```python
from build123d import *
from build123d.topology import SkipClean

# Parameters (mm, degrees)
BOSS_EXTRUDE1_DEPTH      = 3
BOSS_EXTRUDE1_DEPTH_BACK = 1.5
SKETCH1_R                = 8
SKETCH2_W                = 16
SKETCH2_H                = 30
BOSS_EXTRUDE2_DEPTH      = 1.5
CUT_EXTRUDE1_REACH       = 33.373
SKETCH3_R                = 1.25


with BuildPart() as part:
    # Sketch1 → Boss-Extrude1 (new, two sides: drawn at the far end of the back side and taken through both)
    with BuildSketch(Plane(origin=(0, 0, 0), x_dir=(1, 0, 0), z_dir=(0, 1, 0)).offset(-BOSS_EXTRUDE1_DEPTH_BACK)):
        with Locations(Location((0, 0, 0), (0, 0, 270))):
            Circle(SKETCH1_R)
    extrude(amount=BOSS_EXTRUDE1_DEPTH + BOSS_EXTRUDE1_DEPTH_BACK)

    # Sketch2 → Boss-Extrude2 (add, symmetric)
    with BuildSketch(Plane(origin=(0, 0, 0), x_dir=(1, 0, 0), z_dir=(0, 1, 0))):
        with Locations((0, -15)):
            Rectangle(SKETCH2_W, SKETCH2_H)
    extrude(amount=BOSS_EXTRUDE2_DEPTH, both=True)

    # Sketch3 → Cut-Extrude1 (cut, up to next)
    with BuildSketch(Plane(origin=(0, -1.5, 0), x_dir=(-1, 0, 0), z_dir=(0, -1, 0)), mode=Mode.PRIVATE) as cut_extrude1_sk1:
        with Locations(Location((2.503073418, -25.5, 0), (0, 0, 90))):
            Circle(SKETCH3_R)
    cut_extrude1_tool1 = extrude(cut_extrude1_sk1.sketch, amount=-CUT_EXTRUDE1_REACH, mode=Mode.PRIVATE) & part.part
    # Sketch3 → Cut-Extrude1 (cut, up to next)
    with BuildSketch(Plane(origin=(0, -1.5, 0), x_dir=(-1, 0, 0), z_dir=(0, -1, 0)), mode=Mode.PRIVATE) as cut_extrude1_sk2:
        with Locations(Location((-2.503073418, -25.5, 0), (0, 0, 90))):
            Circle(SKETCH3_R)
    cut_extrude1_tool2 = extrude(cut_extrude1_sk2.sketch, amount=-CUT_EXTRUDE1_REACH, mode=Mode.PRIVATE) & part.part
    add(cut_extrude1_tool1.solids().sort_by_distance((-2.503073, -1.5, 25.5))[0], mode=Mode.SUBTRACT)
    add(cut_extrude1_tool2.solids().sort_by_distance((2.503073, -1.5, 25.5))[0], mode=Mode.SUBTRACT)

    # Sketch4 → Cut-Revolve21 (revolve, cut)
    with SkipClean():  # the faces are left unmerged after this step: merging them gives an invalid solid
        with BuildSketch(Plane(origin=(0, -1.5, 0), x_dir=(-1, 0, 0), z_dir=(0, -1, 0))):
            with BuildLine():
                ThreePointArc((3.3, 0), (0, 3.3), (-3.3, 0))
                Line((-3.3, 0), (3.3, 0))
            make_face()
            with BuildLine():
                Line((3.3, 0), (-3.3, 0))
                ThreePointArc((-3.3, 0), (0, -3.3), (3.3, 0))
            make_face()
        revolve(axis=Axis((3.3, -1.5, 0), (-1, 0, 0)), mode=Mode.SUBTRACT)
    add(part.part.scale(1), mode=Mode.REPLACE)  # the faces are merged on a copy


solid = part.part
```
Could you check a few things on this model? Use its own coordinates, in mm. A direction names the side the tool comes from. Give positions to 0.01 mm unless a question says otherwise; leave off trailing zeros. Write each loop counter-clockwise with the first axis right and the second up, starting at its lowest first coordinate (ties: lowest second). Pieces come first, ordered by that corner, then holes. Notation, with made-up numbers: (52.25, 14.5) - (57.25, 14.5) arc R30 ccw to (57.25, 44.5) - close; hole circle Ø2 at (49, 16). An arc over 180 degrees is marked (long way). One line per item, written item: value. Start each with the question number.
Item 1: Imagine slicing it at B-B, the plane y = -0.3. List the corners of the cut face in (x, z) for me, and give its area (3 significant figures).
Item 2: If we mould it in two halves opening along X, with no side actions, what happens to faces 3 (the face through (-8, 0, 15)), 4 (the face through (0, 0, 30)), 5 (the face through (-2.982, -0.021, 24.345))? For each: +X half, -X half, draft (parallel to the pull), parting line (faces both ways), or undercut.
Item 3: Which directions (+Z, -Z, +X, -X, +Y, -Y) give clear straight access to the entire face, cutting with the end or side of a thin tool? Please do faces 1 (the face through (0, 1, -8)), 2 (the face through (8, 0, 15)).
Item 4: Please list where these lines run through material, in increasing order: line 1 (X direction, y = -0.65, z = 25.5); line 2 (X direction, y = 1.2, z = 26.5); line 3 (Y direction, x = -0.5, z = 16). Write a range as from..to.
Item 5: Imagine slicing it at A-A, the plane z = 25.5. List the corners of the cut face in (x, y) for me, and give its area (3 significant figures).
Item 6: Imagine slicing it at D-D, the plane z = 18.5. List the corners of the cut face in (x, y) for me, and give its area (3 significant figures).
Item 7: I'm going to push flat-ended pins straight in: pin 1 (1.5 mm diameter, centred on x = -2.5, z = 25.5, fed in from +Y); pin 2 (8 mm diameter, centred on x = -1, z = 18, fed in from +Y). Where does each tip first touch, or does it pass through?
Item 8: Imagine slicing it at C-C, the plane x = 0. List the corners of the cut face in (y, z) for me.
Geometry says:
1. outline: (-8, 0) arc R8 ccw to (8, 0) - (8, 30) - (-8, 30) - close; hole circle Ø2.5 at (-2.5, 25.5); hole circle Ø6.15 at (0, 0); hole circle Ø2.5 at (2.5, 25.5)
1. area: 541 mm^2
2. face 3: -X half
2. face 4: draft
2. face 5: undercut
3. face 1: +Y
3. face 2: +Z, -Z, +X, +Y, -Y
4. line 1: -8..-3.75, -1.25..1.25, 3.75..8
4. line 2: -8..-3.25, -1.75..1.75, 3.25..8
4. line 3: -1.5..1.5
5. outline: (-8, -1.5) - (-3.75, -1.5) - (-3.75, 1.5) - (-8, 1.5) - close; (-1.25, -1.5) - (1.25, -1.5) - (1.25, 1.5) - (-1.25, 1.5) - close; (3.75, -1.5) - (8, -1.5) - (8, 1.5) - (3.75, 1.5) - close
5. area: 33.0 mm^2
6. outline: (-8, -1.5) - (8, -1.5) - (8, 1.5) - (-8, 1.5) - close
6. area: 48.0 mm^2
7. pin 1: through
7. pin 2: y = 1.5
8. outline: (-1.5, -8) - (3, -8) - (3, 8) - (1.5, 8) - (1.5, 30) - (-1.5, 30) - (-1.5, 3.3) arc R3.3 cw to (-1.5, -3.3) - close
